The listing builds one solid part. Answer for the finished solid, in the listing's coordinates (mm). A direction names the side the tool comes from. Round coordinates to 2 decimals unless told otherwise and drop trailing zeros. Write each loop counter-clockwise with the first axis right and the second up, starting at its lowest first coordinate (ties: lowest second). Pieces come first, ordered by that corner, then holes.
Item 1: Each of these flat-tipped pins is pushed along its axis until it touches: pin 1 (3 mm diameter, centred on y = 0.5, z = 3.5, fed in from -X); pin 2 (5 mm diameter, centred on y = -2.5, z = 8.5, fed in from +X); pin 3 (2 mm diameter, centred on x = 2.5, z = 2.5, fed in from +Y); pin 4 (2 mm diameter, centred on x = 0, z = 6.5, fed in from -Y). Where does it stop, or does it pass through?
Item 2: Find section D-D on x = 5.5. Give the vertices of the cut face in (y, z), then the cut area to 3 significant figures.
Item 3: Find section C-C on x = -2. Give the vertices of the cut face in (y, z).
Item 4: Find section A-A on x = 0. Give the vertices of the cut face in (y, z) (3 decimals), then the cut area to 3 significant figures.
Item 5: A tool of negligible diameter and unlimited length cuts with its end or side. For faces 4 (the face through (0.761, 4.879, 7.964)), 5 (the face through (2, 6, 3)), 6 (the face through (4.88, -0.07, 4.85)), from which of +Z, -Z, +X, -X, +Y, -Y can it reach the whole face along a straight path? Write none if from no direction.
Item 6: Find the intervals of material crossed by probe 1 along Z at (x, y) = (4.8, 0); probe 2 along Y at (x, z) = (0, 2) (3 decimals); probe 3 along Y at (x, z) = (0, 8) (3 decimals), in increasing order.
Item 7: Find section B-B on z = 6.5. Give the vertices of the cut face in (x, y) (3 decimals), then the cut area to 3 significant figures.
Item 8: For a pull along Y with two mould halves and no side action, classify faces 1 (the face through (-3.234, -2.48, 5.07)), 2 (the face through (4, 2, 0)), 3 (the face through (4.57, 7.167, 1.479)) as +Y half, -Y half, draft (parallel to the pull), parting line (faces both ways), or undercut.
```python
from build123d import *

# Parameters (mm, degrees)
SKETCH_2_R                       = 8.5
EXTRUDE_2_DEPTH                  = 3
SKETCH_3_R                       = 6
EXTRUDE_3_DEPTH                  = 7
SKETCH_4_R                       = 4.075
CUT_EXTRUDE_1_DEPTH              = 16.636495771
HOLE_WIZARD_M4_3_REACH           = 20.021
HOLE_WIZARD_M4_3_BORE_R          = 1.65
HOLE_WIZARD_M4_3_ON_FACE_2_REACH = 20.021
HOLE_WIZARD_M4_3_BORE_2_R        = 1.65


with BuildPart() as part:
    # 스케치2 → 보스-돌출2 (new body)
    with BuildSketch(Plane.XY):
        Circle(SKETCH_2_R)
    extrude(amount=EXTRUDE_2_DEPTH)

    # 스케치3 → 보스-돌출3 (add)
    with BuildSketch(Plane.XY.offset(3)):
        Circle(SKETCH_3_R)
    extrude(amount=EXTRUDE_3_DEPTH)

    # 스케치4 → 컷-돌출1 (cut, through all)
    with BuildSketch(Plane.XY.offset(10)):
        Circle(SKETCH_4_R)
    extrude(amount=-CUT_EXTRUDE_1_DEPTH, mode=Mode.SUBTRACT)

    # M4 나사 구멍3 bore (on position points) → M4 나사 구멍3 (cut, up to next)
    with BuildSketch(Plane(origin=(0, 6, 6.5), x_dir=(1, 0, 0), z_dir=(0, 1, 0)), mode=Mode.PRIVATE) as hole_wizard_m4_3_sk1:
        Circle(HOLE_WIZARD_M4_3_BORE_R)
    hole_wizard_m4_3_tool1 = extrude(hole_wizard_m4_3_sk1.sketch, amount=-HOLE_WIZARD_M4_3_REACH, mode=Mode.PRIVATE) & part.part
    add(hole_wizard_m4_3_tool1.solids().sort_by_distance((0, 6, 6.5))[0], mode=Mode.SUBTRACT)

    # M4 나사 구멍3 bore 2 (on position points) → M4 나사 구멍3 on face 2 (cut, up to next)
    with BuildSketch(Plane(origin=(6, 0, 6.5), x_dir=(0, 0, 1), z_dir=(1, 0, 0)), mode=Mode.PRIVATE) as hole_wizard_m4_3_on_face_2_sk1:
        Circle(HOLE_WIZARD_M4_3_BORE_2_R)
    hole_wizard_m4_3_on_face_2_tool1 = extrude(hole_wizard_m4_3_on_face_2_sk1.sketch, amount=-HOLE_WIZARD_M4_3_ON_FACE_2_REACH, mode=Mode.PRIVATE) & part.part
    add(hole_wizard_m4_3_on_face_2_tool1.solids().sort_by_distance((6, 0, 6.5))[0], mode=Mode.SUBTRACT)


solid = part.part
```
Check values:
1. pin 1: stops at x = -8.5
1. pin 2: stops at x = 6
1. pin 3: stops at y = 8.37
1. pin 4: stops at y = -6
2. outline: (-6.48, 0) - (6.48, 0) - (6.48, 3) - (2.4, 3) - (2.4, 10) - (-2.4, 10) - (-2.4, 3) - (-6.48, 3) - close; hole circle Ø3.3 at (0, 6.5)
2. area: 63.9 mm2
3. outline: (-8.26, 0) - (-3.55, 0) - (-3.55, 10) - (-5.66, 10) - (-5.66, 3) - (-8.26, 3) - close; (3.55, 0) - (8.26, 0) - (8.26, 3) - (5.66, 3) - (5.66, 10) - (3.55, 10) - close
4. outline: (-8.5, 0) - (-4.075, 0) - (-4.075, 10) - (-6, 10) - (-6, 3) - (-8.5, 3) - close; (4.075, 0) - (8.5, 0) - (8.5, 3) - (6, 3) - (6, 4.85) - (4.075, 4.85) - close; (4.075, 8.15) - (6, 8.15) - (6, 10) - (4.075, 10) - close
4. area: 47.1 mm2
5. face 4: +Y
5. face 5: +Z
5. face 6: +X
6. probe 1: z = 0 to 4.85, 8.15 to 10
6. probe 2: y = -8.5 to -4.075, 4.075 to 8.5
6. probe 3: y = -6 to -4.075
7. outline: (-1.65, 3.726) - (-1.65, 5.769) arc R6 ccw (long way) to (5.769, -1.65) - (3.726, -1.65) arc R4.075 cw (long way) to start; (1.65, 3.726) arc R4.075 cw to (3.726, 1.65) - (5.769, 1.65) arc R6 ccw to (1.65, 5.769) - close
7. area: 48.0 mm2
8. face 1: undercut
8. face 2: draft
8. face 3: parting line
